Autodesk Inventor part; units mm, degrees
ref_plane "YZ Plane" through (0, 0, 0) normal (1, 0, 0) x (0, 1, 0)
ref_plane "XZ Plane" through (0, 0, 0) normal (0, 1, 0) x (-1, 0, 0)
ref_plane "XY Plane" through (0, 0, 0) normal (0, 0, 1) x (1, 0, 0)
sketch "Sketch1" plane through (0, 0, 0) normal (0, 1, 0) x (-1, 0, 0)
  line L0 (0, 0) -> (6, 0)
  line L1 (6, 0) -> (6, -6)
  line L2 (6, -6) -> (0, -6)
  line L3 (0, -6) -> (0, 0)
  line L4 (0, -6) -> (-55, -6)
  line L5 (-55, -6) -> (-55, 378)
  line L6 (-55, 378) -> (0, 378)
  line L7 (0, 378) -> (0, -6)
  dimension "d0" = 6
  dimension "d1" = 6
  dimension "d2" = 55
  dimension "d3" = 384
extrude "Extrusion1" add sketch "Sketch1" along normal blind 6
mirror "Mirror1" about plane through (55, 0, 378) normal (1, 0, 0) of "Extrusion1"
properties part number "wall 2 for sorting"
Check sheet for the modelled part. Datum: model origin and axes. Units: mm. Coordinates: 2 decimals unless noted, no trailing zeros. Order: outer loops, then holes, each group sorted by start corner. A loop starts at its lowest first (then second) coordinate and runs counter-clockwise, first axis right, second up. Notation, with made-up numbers: (75.25, 14) -> (85.25, 14) arc R9 cw to (85.25, 21) -> close; hole circle Ø4 at (75, 56.5). An arc over 180 degrees is marked (long way). Write item = value, one per line. Start each with the question number.
1) Cross-section at A-A (y = 2.05). Enter the section's corners in (x, z).
2) Cross-section at B-B (z = 36.5). Enter the section's corners in (x, y).
3) Material ranges on L1, parallel to X at y = 4.55, z = 270.5, recorded low to high.
4) Go/stop test with flat-tipped pins: P1, Ø1.8, axis at y = 2, z = 271.5, coming from the +X side; P2, Ø3, axis at x = -4.5, y = 3.5, coming from the +Z side; P3, Ø3, axis at y = 2.5, z = 141, coming from the -X side. Record where each tip stops, or that it passes through.
Ans:
q1.outline = (-6, -6) -> (116, -6) -> (116, 0) -> (110, 0) -> (110, 378) -> (0, 378) -> (0, 0) -> (-6, 0) -> close
q2.outline = (0, 0) -> (110, 0) -> (110, 6) -> (0, 6) -> close
q3.L1 = 0 to 110
q4.P1 = 110
q4.P2 = 0
q4.P3 = 0
